from build123d import *

# Parameters (mm, degrees)
SKIZZE1_R                       = 1.05
AUFSATZ_LINEAR_AUSTRAGEN1_DEPTH = 2
SCHNITT_LINEAR_AUSTRAGEN1_DEPTH = 0.3
SCHNITT_LINEAR_AUSTRAGEN2_REACH = 36.592


with BuildPart() as part:
    # Skizze1 → Aufsatz-Linear austragen1 (new body)
    with BuildSketch(Plane(origin=(0, 0, 0), x_dir=(0, 1, 0), z_dir=(0, 0, 1))):
        with BuildLine():
            Line((-16.65, 7.5), (-16.65, -7.5))
            ThreePointArc((-16.65, -7.5), (-16.166726189, -8.666726189), (-15, -9.15))
            Line((-15, -9.15), (15, -9.15))
            ThreePointArc((15, -9.15), (16.166726189, -8.666726189), (16.65, -7.5))
            Line((16.65, -7.5), (16.65, 7.5))
            ThreePointArc((16.65, 7.5), (16.166726189, 8.666726189), (15, 9.15))
            Line((15, 9.15), (-15, 9.15))
            ThreePointArc((-15, 9.15), (-16.166726189, 8.666726189), (-16.65, 7.5))
        make_face()
        with Locations(Location((-15, 7.5, 0), (0, 0, 270))):
            Circle(SKIZZE1_R, mode=Mode.SUBTRACT)
        with Locations(Location((15, 7.5, 0), (0, 0, 270))):
            Circle(SKIZZE1_R, mode=Mode.SUBTRACT)
        with Locations(Location((15, -7.5, 0), (0, 0, 270))):
            Circle(SKIZZE1_R, mode=Mode.SUBTRACT)
        with Locations(Location((-15, -7.5, 0), (0, 0, 270))):
            Circle(SKIZZE1_R, mode=Mode.SUBTRACT)
        with BuildLine():
            Line((-14.5, 2.5), (-14.5, -2.5))
            ThreePointArc((-14.5, -2.5), (-13.181980515, -5.681980515), (-10, -7))
            Line((-10, -7), (10, -7))
            ThreePointArc((10, -7), (13.181980515, -5.681980515), (14.5, -2.5))
            Line((14.5, -2.5), (14.5, 2.5))
            ThreePointArc((14.5, 2.5), (13.181980515, 5.681980515), (10, 7))
            Line((10, 7), (-10, 7))
            ThreePointArc((-10, 7), (-13.181980515, 5.681980515), (-14.5, 2.5))
        make_face(mode=Mode.SUBTRACT)
    extrude(amount=AUFSATZ_LINEAR_AUSTRAGEN1_DEPTH)

    # Skizze2 → Schnitt-Linear austragen1 (cut)
    with BuildSketch(Plane.XY.offset(2)):
        with BuildLine():
            Line((-2.5, -15.1), (2.5, -15.1))
            ThreePointArc((2.5, -15.1), (6.106244584, -13.606244584), (7.6, -10))
            Line((7.6, -10), (7.6, 10))
            ThreePointArc((7.6, 10), (6.106244584, 13.606244584), (2.5, 15.1))
            Line((2.5, 15.1), (-2.5, 15.1))
            ThreePointArc((-2.5, 15.1), (-6.106244584, 13.606244584), (-7.6, 10))
            Line((-7.6, 10), (-7.6, -10))
            ThreePointArc((-7.6, -10), (-6.106244584, -13.606244584), (-2.5, -15.1))
        make_face()
    extrude(amount=-SCHNITT_LINEAR_AUSTRAGEN1_DEPTH, mode=Mode.SUBTRACT)

    # Schnitt-Linear austragen2: up to this face of the body (flat: up to its plane)
    schnitt_linear_austragen2_end = Plane(part.part.faces().sort_by_distance((0, 16.65, 1))[0])
    # Skizze3 → Schnitt-Linear austragen2 (cut, up to the picked face)
    with BuildSketch(Plane.XZ.offset(16.65), mode=Mode.PRIVATE) as schnitt_linear_austragen2_sk1:
        with BuildLine():
            Line((-1.75, 2), (1.75, 2))
            ThreePointArc((1.75, 2), (0, 0.25), (-1.75, 2))
        make_face()
    schnitt_linear_austragen2_tool1 = split(extrude(schnitt_linear_austragen2_sk1.sketch, amount=-SCHNITT_LINEAR_AUSTRAGEN2_REACH, mode=Mode.PRIVATE), bisect_by=schnitt_linear_austragen2_end, keep=Keep.BOTH, mode=Mode.PRIVATE)
    add(schnitt_linear_austragen2_tool1.solids().sort_by(Axis((0, -16.65, 1.257277), (0, 1, 0)))[0], mode=Mode.SUBTRACT)


solid = part.part
Source: CAD feature listing. Evaluate the final solid. Frame: model axes, mm. A direction names the side the tool comes from. Round coordinates to 2 decimals unless told otherwise and drop trailing zeros. Loops run counter-clockwise (first coordinate to the right, second up) from the corner with the lowest first, then second, coordinate; pieces in that order, holes last. Notation, with made-up numbers: M -31.5,46 L 15.5,46 A20 cw 15.5,71 Z; hole C 63,85 d3. An arc over 180 degrees is marked long. Return JSON: item names as keys, results as strings. Group by question number.
1. Section query B-B on z = 1.2. Output: boundary loops of the cut face in (x, y).
2. Reachability of faces 1 (the face through (-7.5, -0.1, 0)), 2 (the face through (-5.647, 13.217, 0.838)), 3 (the face through (7.3, 1.2, 1.7)) from +Z, -Z, +X, -X, +Y, -Y: full face, straight path, thin tool, end or side. Return the list, or none.
3. Mould query, pull axis X, two halves, no side actions, for faces 4 (the face through (-8.654, 16.179, 0.986)), 5 (the face through (0.04, 15.56, 0.25)), 6 (the face through (8, 0, 2)). Classes: released by +X, released by -X, zero draft, split by the parting line, or undercut.
4. Section query D-D on y = -13. Output: boundary loops of the cut face in (x, z).
5. Material intervals for line 1 along Y through (x, z) = (-7.5, 1.3); line 2 along Y through (x, z) = (2.25, 1.65); line 3 along X through (y, z) = (3, 0.25), sorted ascending. Write a range as from..to.
6. Section query C-C on y = -9.5. Output: boundary loops of the cut face in (x, z).
7. Pin query (flat end, axial travel): pin 1 (3 mm diameter, centred on x = 6, y = -3.5, fed in from +Z). Return the tip coordinate at first contact, or that it passes through.
8. Section query A-A on x = 0. Output: boundary loops of the cut face in (y, z).
Checks:
{
 "1": {"outline": "M -9.15,-15 A1.65 ccw -7.5,-16.65 L -1.56,-16.65 L -1.56,-14.5 L -2.5,-14.5 A4.5 cw -7,-10 L -7,10 A4.5 cw -2.5,14.5 L -1.56,14.5 L -1.56,16.65 L -7.5,16.65 A1.65 ccw -9.15,15 Z; M 1.56,-16.65 L 7.5,-16.65 A1.65 ccw 9.15,-15 L 9.15,15 A1.65 ccw 7.5,16.65 L 1.56,16.65 L 1.56,14.5 L 2.5,14.5 A4.5 cw 7,10 L 7,-10 A4.5 cw 2.5,-14.5 L 1.56,-14.5 Z; hole C -7.5,-15 d2.1; hole C -7.5,15 d2.1; hole C 7.5,-15 d2.1; hole C 7.5,15 d2.1"},
 "2": {"face 1": "-Z, +X, -X, +Y, -Y", "face 2": "+Z, -Z", "face 3": "+Z"},
 "3": {"face 4": "released by -X", "face 5": "undercut", "face 6": "zero draft"},
 "4": {"outline": "M -9.15,0 L -5.85,0 L -5.85,1.7 L -6.62,1.7 L -6.62,2 L -9.15,2 Z; M 5.85,0 L 9.15,0 L 9.15,2 L 6.62,2 L 6.62,1.7 L 5.85,1.7 Z"},
 "5": {"line 1": "y = -16.65..-16.05, -13.95..13.95, 16.05..16.65", "line 2": "y = -16.65..-14.5, 14.5..16.65", "line 3": "x = -9.15..-7, 7..9.15"},
 "6": {"outline": "M -9.15,0 L -7,0 L -7,1.7 L -7.6,1.7 L -7.6,2 L -9.15,2 Z; M 7,0 L 9.15,0 L 9.15,2 L 7.6,2 L 7.6,1.7 L 7,1.7 Z"},
 "7": {"pin 1": "stops at z = 1.7"},
 "8": {"outline": "M -16.65,0 L -14.5,0 L -14.5,0.25 L -16.65,0.25 Z; M 14.5,0 L 16.65,0 L 16.65,0.25 L 14.5,0.25 Z"}
}
